Read the model definition and answer for the solid it produces. Units are mm, in the model's axes. Round coordinates to 2 decimals unless told otherwise and drop trailing zeros. Write each loop counter-clockwise with the first axis right and the second up, starting at its lowest first coordinate (ties: lowest second). Pieces come first, ordered by that corner, then holes. Notation, with made-up numbers: (22.5, 29.25) - (76.5, 29.25) arc R14 ccw to (76.5, 44.25) - close; hole circle Ø2 at (66.5, 37.5). An arc over 180 degrees is marked (long way). Answer as CSV lines item,"result". Start each with the question number.
1) Consider line 1 along X through (y, z) = (63.5, 2); line 2 along Y through (x, z) = (-91.5, 0.3) (3 decimals); line 3 along X through (y, z) = (121.5, 0.45). Determine where each line is inside the solid, lowest interval first.
2) Find section A-A on z = 2.65. Determine the outline of the cut face in (x, y) (3 decimals), then the cut area to 3 significant figures.
3) Each of these flat-tipped pins is pushed along its axis until it touches: pin 1 (1 mm diameter, centred on x = -30, z = 1.5, fed in from -Y) (3 decimals); pin 2 (4 mm diameter, centred on x = -78, y = 722, fed in from -Z). Where does it stop, or does it pass through?
4) Find section C-C on y = 752. Determine the outline of the cut face in (x, z) (1 decimal).
5) Find section B-B on x = -86. Determine the outline of the cut face in (y, z) (3 decimals).
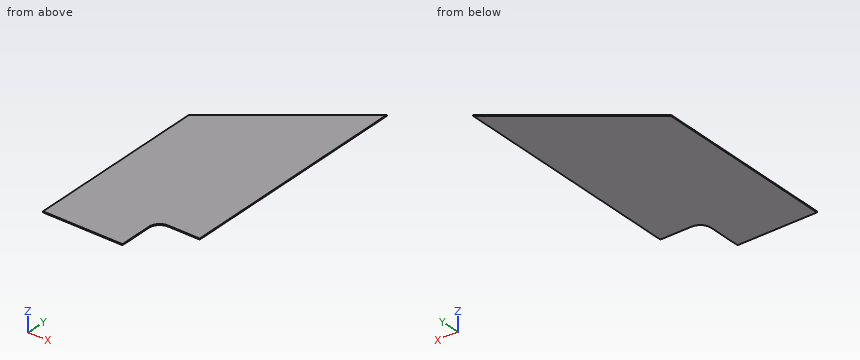
from build123d import *

# Parameters (mm, degrees)
BOSS_EXTRUDE1_DEPTH = 3.175
CUT_EXTRUDE3_DEPTH  = 4.175


with BuildPart() as part:
    # Sketch1 → Boss-Extrude1 (new body)
    with BuildSketch(Plane.XY):
        Polygon((0, 0), (-393.7, 0), (-393.7, 596.9), (0, 908.942774901), align=None)
    extrude(amount=BOSS_EXTRUDE1_DEPTH)

    # Sketch4 → Cut-Extrude3 (cut, through all)
    with BuildSketch(Plane.XY.offset(3.175)):
        with BuildLine():
            Line((0, 0), (-136.652, 0))
            Line((-136.652, 0), (-136.652, 107.95))
            ThreePointArc((-136.652, 107.95), (-126.422704333, 132.645704333), (-101.727, 142.875))
            Line((-101.727, 142.875), (0, 142.875))
            Line((0, 142.875), (0, 0))
        make_face()
    extrude(amount=-CUT_EXTRUDE3_DEPTH, mode=Mode.SUBTRACT)


solid = part.part
Check values:
1,line 1,"x = -393.7 to -136.65"
1,line 2,"y = 142.875 to 836.421"
1,line 3,"x = -393.7 to -133.92"
2,outline,"(-393.7, 0) - (-136.652, 0) - (-136.652, 107.95) arc R34.925 cw to (-101.727, 142.875) - (0, 142.875) - (0, 908.943) - (-393.7, 596.9) - close"
2,area,"277,000 mm^2"
3,pin 1,"stops at y = 142.875"
3,pin 2,"stops at z = 0"
4,outline,"(-198, 0) - (0, 0) - (0, 3.2) - (-198, 3.2) - close"
5,outline,"(142.875, 0) - (840.78, 0) - (840.78, 3.175) - (142.875, 3.175) - close"
